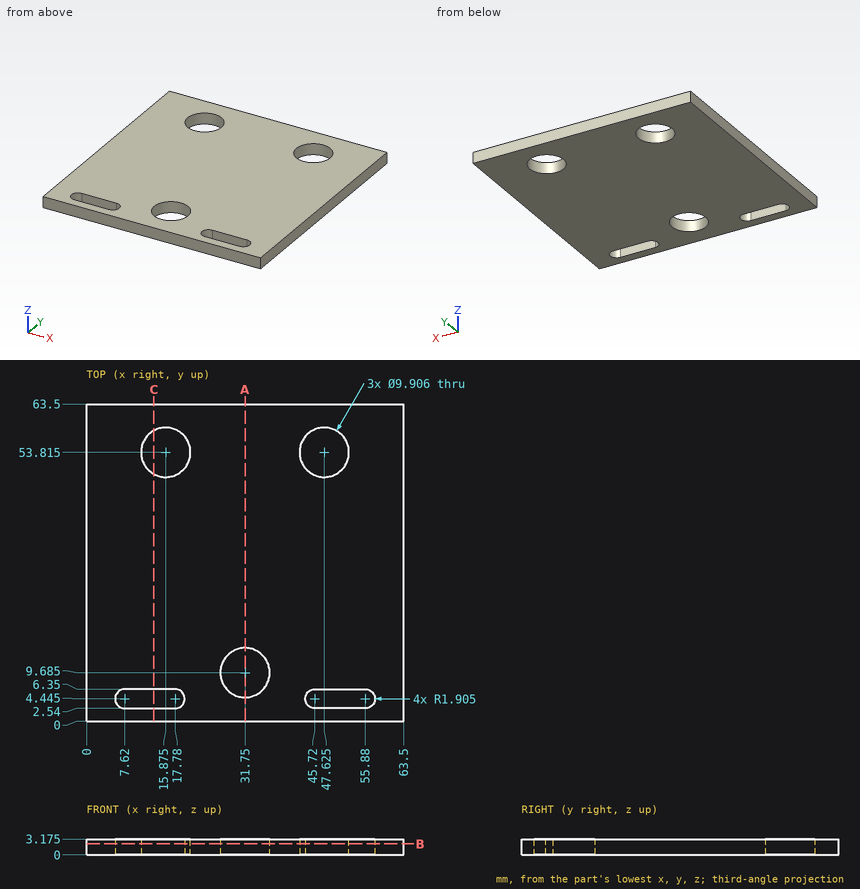
Source: three-view drawing plus pictorial views. Frame: mm from the lowest corner of the part. Coordinates: 2 decimals unless noted, no trailing zeros. Write each loop counter-clockwise with the first axis right and the second up, starting at its lowest first coordinate (ties: lowest second). Pieces come first, ordered by that corner, then holes. Notation, with made-up numbers: (49.5, -6) -> (82.5, -6) arc R14 ccw to (82.5, 7) -> close; hole circle Ø11 at (-29, -11.5). An arc over 180 degrees is marked (long way). Write each question's results on one line, items separated by ' | '.
Item 1: Section query A-A on x = 31.75. Return loops of the section in (y, z) (3 decimals), plus the area to 3 significant figures.
Conclusion:
outline: (0, 0) -> (4.732, 0) -> (4.732, 3.175) -> (0, 3.175) -> close; (14.638, 0) -> (63.5, 0) -> (63.5, 3.175) -> (14.638, 3.175) -> close | area: 170 mm^2
Item 2: Section query C-C on x = 13.5. Count the separate pieces of the cut face and the enclosed holes in it, plus the area to 3 significant figures.
Conclusion:
separate pieces: 3 | enclosed holes: 0 | area: 162 mm^2
Item 3: Material intervals for probe 1 along Y at (x, z) = (10, 2.35); probe 2 along Y at (x, z) = (48.5, 0.75); probe 3 along Y at (x, z) = (31.75, 1.8), sorted ascending.
Conclusion:
probe 1: y = 0 to 2.54, 6.35 to 63.5 | probe 2: y = 0 to 2.54, 6.35 to 48.94, 58.69 to 63.5 | probe 3: y = 0 to 4.73, 14.64 to 63.5
Item 4: Pin query (flat end, axial travel): pin 1 Ø1.6 at (x, z) = (52, 1) entering from -Y; pin 2 Ø6 at (x, y) = (31.75, 9.69) entering from -Z. Return the tip coordinate at first contact, or that it passes through.
Conclusion:
pin 1: stops at y = 0 | pin 2: passes through
Item 5: Section query B-B on z = 2.2. Return loops of the section in (x, y) (3 decimals), plus the area to 3 significant figures.
Conclusion:
outline: (0, 0) -> (63.5, 0) -> (63.5, 63.5) -> (0, 63.5) -> close; hole (7.62, 2.54) -> (17.78, 2.54) arc R1.905 ccw to (17.78, 6.35) -> (7.62, 6.35) arc R1.905 ccw to start; hole circle Ø9.906 at (15.875, 53.815); hole circle Ø9.906 at (31.75, 9.685); hole circle Ø9.906 at (47.625, 53.815); hole (45.72, 2.54) -> (55.88, 2.54) arc R1.905 ccw to (55.88, 6.35) -> (45.72, 6.35) arc R1.905 ccw to start | area: 3,700 mm^2
